Geometry: final body of the model. Coordinates: model frame, mm. A direction names the side the tool comes from. Round coordinates to 2 decimals unless told otherwise and drop trailing zeros. Write each loop counter-clockwise with the first axis right and the second up, starting at its lowest first coordinate (ties: lowest second). Pieces come first, ordered by that corner, then holes. Notation, with made-up numbers: M -35,-29.5 L -1,-29.5 A25 cw -1,8.5 Z; hole C 85,23 d1. An arc over 180 degrees is marked long. Answer as CSV lines item,"result". Start each with the question number.
Q1. Ray query, probe 1 along Z at (x, y) = (12, -36); probe 2 along X at (y, z) = (-0.5, 71) (3 decimals); probe 3 along Y at (x, z) = (0, 34). Return the intervals inside material, ascending.
Q2. First-contact query: pin 1 (5 mm diameter, centred on y = 21.5, z = 67.5, fed in from +X); pin 2 (2 mm diameter, centred on x = 5.5, y = -71.5, fed in from -Z); pin 3 (1 mm diameter, centred on y = 59, z = 87.5, fed in from -X). Flat tips, straight axial feed; report the tip coordinate or a pass-through.
Q3. Reachability of faces 1 (the cylindrical face through (26.566, 89.474, 1.014)), 2 (the cylindrical face through (-26.57, 89.47, 87.01)) from +Z, -Z, +X, -X, +Y, -Y: full face, straight path, thin tool, end or side. Return the list, or none.
Q4. Section query A-A on z = 17. Output: boundary loops of the cut face in (x, y).
Q5. Mould query, pull axis Y, two halves, no side actions, for faces 3 (the flat face through (-22, -14, 0)), 4 (the cylindrical face through (-26.566, -89.474, 1.014)). Classes: pulls with the +Y half, pulls with the -Y half, needs draft (parallel to the pull), parting line crosses it, or undercut.
```python
from build123d import *

# Parameters (mm, degrees)
SKICA1_R                 = 100
SKICA1_R_2               = 25
P_IDAT_VYSUNUT_M1_DEPTH  = 88
ODEBRAT_START            = -80
SKICA2_R                 = 100
SKICA2_R_2               = 35.288223769
ODEBRAT_VYSUNUT_M1_DEPTH = 80
ZAOBLIT1_R               = 1
ODEBRAT_VYSUNUT_M2_DEPTH = 2
ODEBRAT_START_2          = -2
ODEBRAT_VYSUNUT_M3_DEPTH = 2


with BuildPart() as part:
    # Skica1 → Přidat vysunutím1 (new body)
    with BuildSketch(Plane.XY):
        Circle(SKICA1_R)
        Circle(SKICA1_R_2, mode=Mode.SUBTRACT)
    extrude(amount=P_IDAT_VYSUNUT_M1_DEPTH)

    # Skica2 → Odebrat vysunutím1 (cut)
    with BuildSketch(Plane.XY.offset(84).offset(ODEBRAT_START)):
        Circle(SKICA2_R)
        Circle(SKICA2_R_2, mode=Mode.SUBTRACT)
    extrude(amount=ODEBRAT_VYSUNUT_M1_DEPTH, mode=Mode.SUBTRACT)

    # Zaoblit1
    zaoblit1_edges = [part.edges().sort_by_distance(p)[0] for p in [
        (-100, 0, 4),
        (-100, 0, 84),
        (-100, 0, 0),
        (-100, 0, 88),
    ]]
    fillet(zaoblit1_edges, radius=ZAOBLIT1_R)

    # Skica3 → Odebrat vysunutím2 (cut)
    with BuildSketch(Plane.XY.offset(88)):
        with BuildLine():
            Line((0, 35), (0, 93.333333333))
            ThreePointArc((0, 93.333333333), (-26.932410451, 89.363059361), (-51.573484154, 77.790017633))
            Line((-51.573484154, 77.790017633), (-19.340056558, 29.171256612))
            ThreePointArc((-19.340056558, 29.171256612), (-10.099653919, 33.51114726), (0, 35))
        make_face()
        with BuildLine():
            Line((-20.57248383, 28.315594803), (-54.859956881, 75.508252808))
            ThreePointArc((-54.859956881, 75.508252808), (-74.315066147, 56.465760021), (-87.44765028, 32.619312862))
            Line((-87.44765028, 32.619312862), (-32.792868855, 12.232242323))
            ThreePointArc((-32.792868855, 12.232242323), (-27.868149805, 21.174660008), (-20.57248383, 28.315594803))
        make_face()
        with BuildLine():
            ThreePointArc((54.859956881, 75.508252808), (30.737510638, 88.126707364), (4, 93.247579653))
            Line((4, 93.247579653), (1.5, 34.96784237))
            ThreePointArc((1.5, 34.96784237), (11.526566489, 33.047515262), (20.57248383, 28.315594803))
            Line((20.57248383, 28.315594803), (54.859956881, 75.508252808))
        make_face()
        with BuildLine():
            ThreePointArc((88.765274854, 28.841586142), (76.666747393, 53.228948471), (58.045620109, 73.087735614))
            Line((58.045620109, 73.087735614), (21.767107541, 27.407900855))
            ThreePointArc((21.767107541, 27.407900855), (28.750030272, 19.960855677), (33.28697807, 10.815594803))
            Line((33.28697807, 10.815594803), (88.765274854, 28.841586142))
        make_face()
        with BuildLine():
            ThreePointArc((93.333333333, 0), (92.476009032, 12.621365401), (89.919786235, 25.010860732))
            Line((89.919786235, 25.010860732), (33.719919838, 9.379072774))
            ThreePointArc((33.719919838, 9.379072774), (34.678503387, 4.733012025), (35, 0))
            ThreePointArc((35, 0), (34.569091921, -5.475206276), (33.28697807, -10.815594803))
            Line((33.28697807, -10.815594803), (88.765274854, -28.841586142))
            ThreePointArc((88.765274854, -28.841586142), (92.184245122, -14.60055007), (93.333333333, 0))
        make_face()
        with BuildLine():
            ThreePointArc((54.859956881, -75.508252808), (74.315066147, -56.465760021), (87.44765028, -32.619312862))
            Line((87.44765028, -32.619312862), (32.792868855, -12.232242323))
            ThreePointArc((32.792868855, -12.232242323), (27.868149805, -21.174660008), (20.57248383, -28.315594803))
            Line((20.57248383, -28.315594803), (54.859956881, -75.508252808))
        make_face()
        with BuildLine():
            ThreePointArc((0, -93.333333333), (26.932410451, -89.363059361), (51.573484154, -77.790017633))
            Line((51.573484154, -77.790017633), (19.340056558, -29.171256612))
            ThreePointArc((19.340056558, -29.171256612), (10.099653919, -33.51114726), (0, -35))
            Line((0, -35), (0, -93.333333333))
        make_face()
        with BuildLine():
            Line((-20.57248383, -28.315594803), (-54.859956881, -75.508252808))
            ThreePointArc((-54.859956881, -75.508252808), (-30.737510638, -88.126707364), (-4, -93.247579653))
            Line((-4, -93.247579653), (-1.5, -34.96784237))
            ThreePointArc((-1.5, -34.96784237), (-11.526566489, -33.047515262), (-20.57248383, -28.315594803))
        make_face()
        with BuildLine():
            Line((-33.28697807, -10.815594803), (-88.765274854, -28.841586142))
            ThreePointArc((-88.765274854, -28.841586142), (-76.666747393, -53.228948471), (-58.045620109, -73.087735614))
            Line((-58.045620109, -73.087735614), (-21.767107541, -27.407900855))
            ThreePointArc((-21.767107541, -27.407900855), (-28.750030272, -19.960855677), (-33.28697807, -10.815594803))
        make_face()
        with BuildLine():
            Line((-33.28697807, 10.815594803), (-88.765274854, 28.841586142))
            ThreePointArc((-88.765274854, 28.841586142), (-93.31189245, 2.000459553), (-89.919786235, -25.010860732))
            Line((-89.919786235, -25.010860732), (-33.719919838, -9.379072774))
            ThreePointArc((-33.719919838, -9.379072774), (-34.991959669, 0.750172332), (-33.28697807, 10.815594803))
        make_face()
    extrude(amount=-ODEBRAT_VYSUNUT_M2_DEPTH, mode=Mode.SUBTRACT)

    # Skica4 → Odebrat vysunutím3 (cut)
    with BuildSketch(Plane(origin=(0, 0, 0), x_dir=(-1, 0, 0), z_dir=(0, 0, -1)).offset(ODEBRAT_START_2)):
        with BuildLine():
            ThreePointArc((-19.340078903, 29.171241798), (-10.099666754, 33.511143392), (0, 35))
            Line((0, 35), (0, 93.335))
            ThreePointArc((0, 93.335), (-26.932925613, 89.364644815), (-51.574464697, 77.791367234))
            Line((-51.574464697, 77.791367234), (-19.340078903, 29.171241798))
        make_face()
        with BuildLine():
            ThreePointArc((-32.792878225, 12.232217204), (-27.868157915, 21.174649334), (-20.57248383, 28.315594803))
            Line((-20.57248383, 28.315594803), (-54.860936523, 75.50960117))
            ThreePointArc((-54.860936523, 75.50960117), (-74.316414828, 56.466739875), (-87.449236832, 32.619828364))
            Line((-87.449236832, 32.619828364), (-32.792878225, 12.232217204))
        make_face()
        with BuildLine():
            ThreePointArc((-33.719912654, -9.379098604), (-34.991959956, 0.750158931), (-33.28697807, 10.815594803))
            Line((-33.28697807, 10.815594803), (-88.766859948, 28.84210117))
            ThreePointArc((-88.766859948, 28.84210117), (-93.3135595, 2.000459537), (-89.921372787, -25.011376234))
            Line((-89.921372787, -25.011376234), (-33.719912654, -9.379098604))
        make_face()
        with BuildLine():
            ThreePointArc((-21.767086547, -27.407917529), (-28.750022627, -19.960866688), (-33.28697807, -10.815594803))
            Line((-33.28697807, -10.815594803), (-88.766859948, -28.84210117))
            ThreePointArc((-88.766859948, -28.84210117), (-76.668096055, -53.229928352), (-58.046600652, -73.089085216))
            Line((-58.046600652, -73.089085216), (-21.767086547, -27.407917529))
        make_face()
        with BuildLine():
            ThreePointArc((-1.499973215, -34.967843519), (-11.526553832, -33.047519676), (-20.57248383, -28.315594803))
            Line((-20.57248383, -28.315594803), (-54.860936523, -75.50960117))
            ThreePointArc((-54.860936523, -75.50960117), (-30.738025769, -88.128292828), (-4, -93.249247852))
            Line((-4, -93.249247852), (-1.499973215, -34.967843519))
        make_face()
        with BuildLine():
            Line((51.574464697, -77.791367234), (19.340078903, -29.171241798))
            ThreePointArc((19.340078903, -29.171241798), (10.099666754, -33.511143392), (0, -35))
            Line((0, -35), (0, -93.335))
            ThreePointArc((0, -93.335), (26.932925613, -89.364644815), (51.574464697, -77.791367234))
        make_face()
        with BuildLine():
            Line((87.449236832, -32.619828364), (32.792878225, -12.232217204))
            ThreePointArc((32.792878225, -12.232217204), (27.868157915, -21.174649334), (20.57248383, -28.315594803))
            Line((20.57248383, -28.315594803), (54.860936523, -75.50960117))
            ThreePointArc((54.860936523, -75.50960117), (74.316414828, -56.466739875), (87.449236832, -32.619828364))
        make_face()
        with BuildLine():
            Line((89.921372787, 25.011376234), (33.719912654, 9.379098604))
            ThreePointArc((33.719912654, 9.379098604), (34.678501574, 4.733025307), (35, 0))
            ThreePointArc((35, 0), (34.569091921, -5.475206276), (33.28697807, -10.815594803))
            Line((33.28697807, -10.815594803), (88.766859948, -28.84210117))
            ThreePointArc((88.766859948, -28.84210117), (92.185891269, -14.600810795), (93.335, 0))
            ThreePointArc((93.335, 0), (92.477655555, 12.621626201), (89.921372787, 25.011376234))
        make_face()
        with BuildLine():
            Line((58.046600652, 73.089085216), (21.767086547, 27.407917529))
            ThreePointArc((21.767086547, 27.407917529), (28.750022627, 19.960866688), (33.28697807, 10.815594803))
            Line((33.28697807, 10.815594803), (88.766859948, 28.84210117))
            ThreePointArc((88.766859948, 28.84210117), (76.668096055, 53.229928352), (58.046600652, 73.089085216))
        make_face()
        with BuildLine():
            Line((4, 93.249247852), (1.499973215, 34.967843519))
            ThreePointArc((1.499973215, 34.967843519), (11.526553832, 33.047519676), (20.57248383, 28.315594803))
            Line((20.57248383, 28.315594803), (54.860936523, 75.50960117))
            ThreePointArc((54.860936523, 75.50960117), (30.738025769, 88.128292828), (4, 93.249247852))
        make_face()
    extrude(amount=ODEBRAT_VYSUNUT_M3_DEPTH, mode=Mode.SUBTRACT)


solid = part.part
```
Entries:
1,probe 1,"z = 2 to 4, 84 to 86"
1,probe 2,"x = -35.285 to -24.995, 24.995 to 35.285"
1,probe 3,"y = -35.29 to -25, 25 to 35.29"
2,pin 1,"stops at x = 29.74"
2,pin 2,"stops at z = 2"
2,pin 3,"stops at x = -81.02"
3,face 1,"-Z"
3,face 2,"+Z"
4,outline,"C 0,0 d70.58; hole C 0,0 d50"
5,face 3,"needs draft"
5,face 4,"undercut"
